Can you work these out from the model? Positions are in its coordinate system, mm. Give positions to 0.01 mm unless a question says otherwise; leave off trailing zeros. Write each loop counter-clockwise with the first axis right and the second up, starting at its lowest first coordinate (ties: lowest second). Pieces come first, ordered by that corner, then holes.
1. Suppose I cut it at B-B (x = 38). Please give me the cut outline in (y, z) (3 decimals), and give its area (3 significant figures).
2. Suppose I cut it at C-C (z = 2.3). Give the number of separate pieces and of enclosed holes in the cut face, and give its area (3 significant figures).
3. If I drill on probe 1 along X at (y, z) = (51, 2.6) (3 decimals); probe 2 along Y at (x, z) = (111, 2.65), over which ranges is the centre line in solid material (lowest first)?
4. I'm going to push flat-ended pins straight in: pin 1 (1 mm diameter, centred on x = 248, z = 1.5, fed in from -Y) (3 decimals); pin 2 (1.6 mm diameter, centred on x = 79, z = 2, fed in from -Y); pin 3 (2 mm diameter, centred on x = 166.69, y = 4.76, fed in from -Z). Where does each tip first touch, or does it pass through?
5. Suppose I cut it at A-A (y = 42). Please give me the cut outline in (x, z) (3 decimals).
```python
from build123d import *

# Parameters (mm, degrees)
F0_R     = 1.7272
F1_DEPTH = 3.175


with BuildPart() as f1:
    # F0 (on Top) → F1 (new body)
    with BuildSketch(Plane.XY):
        Polygon((0, 0), (0, 76.2), (161.925, 76.2), (161.925, 0), (171.45, 0), (171.45, 9.525), (180.975, 9.525), (180.975, 0), (244.475, 0), (244.475, 9.525), (254, 9.525), (254, 0), (263.525, 0), (263.525, 304.8), (254, 304.8), (254, 295.275), (244.475, 295.275), (244.475, 304.8), (-184.15, 304.8), (-184.15, 295.275), (-193.675, 295.275), (-193.675, 304.8), (-203.2, 304.8), (-203.2, 0), (-193.675, 0), (-193.675, 9.525), (-184.15, 9.525), (-184.15, 0), (-19.05, 0), (-19.05, 9.525), (-9.525, 9.525), (-9.525, 0), align=None)
        with Locations((-198.4375, 4.7625)):
            Circle(F0_R, mode=Mode.SUBTRACT)
        with Locations((-4.7625, 4.7625)):
            Circle(F0_R, mode=Mode.SUBTRACT)
        with Locations((166.6875, 4.7625)):
            Circle(F0_R, mode=Mode.SUBTRACT)
        with Locations((258.7625, 4.7625)):
            Circle(F0_R, mode=Mode.SUBTRACT)
    extrude(amount=F1_DEPTH)


solid = f1.part
```
Checks:
1. outline: (76.2, 0) - (304.8, 0) - (304.8, 3.175) - (76.2, 3.175) - close
1. area: 726 mm2
2. separate pieces: 1
2. enclosed holes: 4
2. area: 129,000 mm2
3. probe 1: x = -203.2 to 0, 161.925 to 263.525
3. probe 2: y = 76.2 to 304.8
4. pin 1: stops at y = 9.525
4. pin 2: stops at y = 76.2
4. pin 3: passes through
5. outline: (-203.2, 0) - (0, 0) - (0, 3.175) - (-203.2, 3.175) - close; (161.925, 0) - (263.525, 0) - (263.525, 3.175) - (161.925, 3.175) - close
